Source: CAD feature listing. Evaluate the final solid. Frame: model axes, mm. Round coordinates to 2 decimals unless told otherwise and drop trailing zeros. Order: outer loops, then holes, each group sorted by start corner. A loop starts at its lowest first (then second) coordinate and runs counter-clockwise, first axis right, second up. Notation, with made-up numbers: (47, 65) - (81, 65) arc R18 ccw to (81, 71) - close; hole circle Ø1 at (7.5, 57). An arc over 180 degrees is marked (long way). Use one line per item in the form item = value. Start each with the question number.
Q1. Draft query along X for faces 1 (the cylindrical face through (11.99, 2.03, -18.15)), 2 (the cylindrical face through (9.1, 2, -11.2)), 3 (the flat face through (-5, 2, 21)). Return one class per face: released by +X, released by -X, zero draft, split by the parting line, or undercut.
Q2. Cut plane A-A, the plane x = 0. Return the cut outline in (y, z), and give its area (3 significant figures).
Q3. Cut plane C-C, the plane y = 0.9. Return the cut outline in (x, z).
Q4. Ray query, line 1 (X direction, y = 2.5, z = 10); line 2 (Z direction, x = -10.25, y = 2.65); line 3 (X direction, y = 1, z = 9.5). Return the intervals inside material, ascending. Write a range as [from, to].
Q5. Cut plane D-D, the plane z = 0. Return the cut outline in (x, y), and give its area (3 significant figures).
Q6. Cut plane B-B, the plane x = -10. Return the cut outline in (y, z).
Q7. Pin query (flat end, axial travel): pin 1 Ø13 at (x, z) = (0, 0) entering from -Y. Return the tip coordinate at first contact, or that it passes through.
from build123d import *

# Parameters (mm, degrees)
SKETCH2_W           = 30
SKETCH2_H           = 42
SKETCH2_R           = 8
BOSS_EXTRUDE1_DEPTH = 4
FILLET1_R           = 10
SKETCH3_R           = 1.5
CUT_EXTRUDE1_DEPTH  = 6


with BuildPart() as part:
    # Sketch2 → Boss-Extrude1 (new body)
    with BuildSketch(Plane(origin=(0, 0, 0), x_dir=(1, 0, 0), z_dir=(0, 1, 0))):
        Rectangle(SKETCH2_W, SKETCH2_H)
        with Locations(Location((0, 0, 0), (0, 0, 270))):
            Circle(SKETCH2_R, mode=Mode.SUBTRACT)
    extrude(amount=BOSS_EXTRUDE1_DEPTH)

    # Fillet1
    fillet1_edges = [part.edges().sort_by_distance(p)[0] for p in [
        (15, 2, 21),
        (15, 2, -21),
    ]]
    fillet(fillet1_edges, radius=FILLET1_R)

    # Sketch3 → Cut-Extrude1 (cut)
    with BuildSketch(Plane(origin=(0, 4, 0), x_dir=(1, 0, 0), z_dir=(0, 1, 0))):
        with Locations(Location((-10, 10, 0), (0, 0, 270))):
            Circle(SKETCH3_R)
        with Locations(Location((10, 10, 0), (0, 0, 270))):
            Circle(SKETCH3_R)
        with Locations(Location((10, -10, 0), (0, 0, 270))):
            Circle(SKETCH3_R)
        with Locations(Location((-10, -10, 0), (0, 0, 270))):
            Circle(SKETCH3_R)
    extrude(amount=-CUT_EXTRUDE1_DEPTH, mode=Mode.SUBTRACT)


solid = part.part
Completed:
q1.face_1 = released by +X
q1.face_2 = undercut
q1.face_3 = zero draft
q2.outline = (0, -21) - (4, -21) - (4, -8) - (0, -8) - close; (0, 8) - (4, 8) - (4, 21) - (0, 21) - close
q2.area = 104 mm2
q3.outline = (-15, -21) - (5, -21) arc R10 ccw to (15, -11) - (15, 11) arc R10 ccw to (5, 21) - (-15, 21) - close; hole circle Ø3 at (-10, -10); hole circle Ø3 at (-10, 10); hole circle Ø16 at (0, 0); hole circle Ø3 at (10, -10); hole circle Ø3 at (10, 10)
q4.line_1 = [-15, -11.5], [-8.5, 8.5], [11.5, 15]
q4.line_2 = [-21, -11.48], [-8.52, 8.52], [11.48, 21]
q4.line_3 = [-15, -11.41], [-8.59, 8.59], [11.41, 15]
q5.outline = (-15, 0) - (-8, 0) - (-8, 4) - (-15, 4) - close; (8, 0) - (15, 0) - (15, 4) - (8, 4) - close
q5.area = 56.0 mm2
q6.outline = (0, -21) - (4, -21) - (4, -11.5) - (0, -11.5) - close; (0, -8.5) - (4, -8.5) - (4, 8.5) - (0, 8.5) - close; (0, 11.5) - (4, 11.5) - (4, 21) - (0, 21) - close
q7.pin_1 = through
